The listing builds one solid part. Answer for the finished solid, in the listing's coordinates (mm). A direction names the side the tool comes from. Coordinates: 2 decimals unless noted, no trailing zeros. Order: outer loops, then holes, each group sorted by start corner. A loop starts at its lowest first (then second) coordinate and runs counter-clockwise, first axis right, second up.
from build123d import *

# Parameters (mm, degrees)
SKETCH007_W          = 124
SKETCH007_H          = 24.5
SKETCH007_R          = 2.5
PAD004_DEPTH         = 2
SKETCH006_R          = 3.175
PAD005_DEPTH         = 4.1125
PAD006_DEPTH         = 12.25
POCKET001_DEPTH      = 373.382623
POCKET001_DEPTH_BACK = 485.092667
PAD007_DEPTH         = 2
SKETCH011_W          = 35
SKETCH011_H          = 30
SKETCH011_W_2        = 15
SKETCH011_H_2        = 17
PAD008_DEPTH         = 12.25
HOLE_D               = 4.5
HOLE_CSINK_D         = 8.8
HOLE_CSINK_ANGLE     = 90
FILLET002_R          = 3
FILLET003_R          = 2
FILLET004_R          = 7
SKETCH017_W          = 3
SKETCH017_H          = 16.275
POCKET004_DEPTH      = 14.161
POCKET004_DEPTH_BACK = 213.001


with BuildPart() as part:
    # Sketch007 → Pad004 (new body)
    with BuildSketch(Plane.XZ.offset(13)):
        with Locations((78, 0)):
            Rectangle(SKETCH007_W, SKETCH007_H)
        with Locations((30, 0)):
            Circle(SKETCH007_R, mode=Mode.SUBTRACT)
        with BuildLine():
            ThreePointArc((90.8685, 2.143), (88.7255, 0), (90.8685, -2.143))
            Line((90.8685, -2.143), (98.806, -2.143))
            ThreePointArc((98.806, -2.143), (100.949, 0), (98.806, 2.143))
            Line((98.806, 2.143), (90.8685, 2.143))
        make_face(mode=Mode.SUBTRACT)
    extrude(amount=PAD004_DEPTH)

    # Sketch006 → Pad005 (join)
    with BuildSketch(Plane.XY.offset(12.25)):
        with BuildLine():
            Line((16, -13), (10.43, -13))
            Line((10.43, -13), (10.43, 3.73))
            ThreePointArc((10.43, 3.73), (2.257465, 13.912767), (-9.45279, 8.137908))
            ThreePointArc((-26.289956, 7.402782), (-17.64833, 2.661824), (-9.45279, 8.137908))
            Line((-26.289956, 7.402782), (-13.355703, -15))
            Line((-13.355703, -15), (16, -15))
            Line((16, -15), (16, -13))
        make_face()
        with Locations((0, 3.73)):
            Circle(SKETCH006_R, mode=Mode.SUBTRACT)
    pad005 = extrude(amount=-PAD005_DEPTH)

    # Mirrored001: Pad005 across XY
    add(pad005.mirror(Plane.XY))

    # Sketch008 → Pad006 (join, symmetric)
    with BuildSketch(Plane.XY):
        Polygon((-26.289956, 7.402782), (-28.289956, 9.134833), (-14.355703, -15), (-13.355703, -15), align=None)
    extrude(amount=PAD006_DEPTH, both=True)

    # Sketch009 → Pocket001 (cut, two sides)
    with BuildSketch(Plane.YZ) as pocket001_sk:
        with BuildLine():
            ThreePointArc((-13, 12.25), (-11.749286, 10.934524), (-10, 10.45))
            Line((-10, 10.45), (14.16, 10.45))
            Line((14.16, 12.25), (14.16, 10.45))
            Line((14.16, 12.25), (-13, 12.25))
        make_face()
    pocket001 = extrude(amount=-POCKET001_DEPTH, mode=Mode.SUBTRACT) + extrude(pocket001_sk.sketch, amount=POCKET001_DEPTH_BACK, mode=Mode.SUBTRACT)

    # Mirrored002: Pocket001 across Sketch009 H_Axis
    add(pocket001.mirror(Plane.XY), mode=Mode.SUBTRACT)

    # Sketch010 → Pad007 (join)
    with BuildSketch(Plane.XY.offset(12.25)):
        with BuildLine():
            Line((-13.355703, -15), (140, -15))
            Line((140, -15), (140, -45))
            Line((11.644297, -45), (140, -45))
            Line((16.00778, -59.929218), (11.644297, -45))
            Line((29.314371, -174.42131), (16.00778, -59.929218))
            Line((35.419102, -190.709129), (29.314371, -174.42131))
            Line((18.174297, -190.709129), (35.419102, -190.709129))
            ThreePointArc((18.174297, -190.709129), (11.242593, -193.580335), (8.371387, -200.512039))
            Line((8.371387, -210.497159), (8.371387, -200.512039))
            Line((-13.355703, -213), (8.371387, -210.497159))
            Line((-13.355703, -213), (-13.355703, -15))
        make_face()
    extrude(amount=-PAD007_DEPTH)

    # Sketch011 (on Face7 of Pad007) → Pad008 (join)
    with BuildSketch(Plane(origin=(0, 0, 12.25), x_dir=(-1, 0, 0), z_dir=(0, 0, 1))):
        with Locations((-36.144297, 30)):
            Rectangle(SKETCH011_W, SKETCH011_H)
        with Locations((-132.5, 36.5)):
            Rectangle(SKETCH011_W_2, SKETCH011_H_2)
        Polygon((13.355703, 174.42131), (-29.314371, 174.42131), (13.355703, 213), align=None)
    extrude(amount=-PAD008_DEPTH)

    # Hole (through all)
    with Locations(Plane.XY.offset(12.25)):
        with Locations((0, -190), (37.5, -30), (132.5, -36.5)):
            CounterSinkHole(HOLE_D / 2, HOLE_CSINK_D / 2, counter_sink_angle=HOLE_CSINK_ANGLE)

    # Fillet002
    fillet002_edges = [part.edges().sort_by_distance(p)[0] for p in [
        (96.822148, -15, 10.25),
    ]]
    fillet(fillet002_edges, radius=FILLET002_R)

    # Fillet003
    fillet003_edges = [part.edges().sort_by_distance(p)[0] for p in [
        (2.644297, -15, 10.25),
    ]]
    fillet(fillet003_edges, radius=FILLET003_R)

    # Fillet004
    fillet004_edges = [part.edges().sort_by_distance(p)[0] for p in [
        (125, -28, 5.125),
        (140, -45, 5.125),
    ]]
    fillet(fillet004_edges, radius=FILLET004_R)

    # Sketch017 → Pocket004 (cut, two sides)
    with BuildSketch(Plane.XZ) as pocket004_sk:
        with Locations((-14.855703, 0)):
            Rectangle(SKETCH017_W, SKETCH017_H)
    extrude(amount=-POCKET004_DEPTH, mode=Mode.SUBTRACT)
    extrude(pocket004_sk.sketch, amount=POCKET004_DEPTH_BACK, mode=Mode.SUBTRACT)


solid = part.part
1) Section B-B (y = -48) is taken. Give the vertices of the cut face in (x, z), then the cut area to 3 significant figures.
2) Section C-C (y = -74) is taken. Give the vertices of the cut face in (x, z).
3) Section A-A (x = 63) is taken. Give the vertices of the cut face in (y, z), then the cut area to 3 significant figures.
4) Consider L1, parallel to Y at x = 0, z = -9.45 (3 decimals); L2, parallel to Y at x = 37.5, z = 4.75; L3, parallel to Y at x = 0, z = 9.8 (3 decimals). Determine where each line is inside the solid, lowest interval first.
5) Determine the mould class of faces 6 (the face through (127.1, -30, 5.1)), 7 (the face through (137.9, -43, 6.2)), 8 (the face through (-4, -1, -10.45)) for opening direction Y: released by +Y, released by -Y, zero draft, split by the parting line, or undercut.
6) Each of these flat-tipped pins is pushed along its axis until it touches: P1, Ø0.6, axis at y = -14, z = -0.5, coming from the -X side; P2, Ø19.5, axis at x = 5.5, y = -191, coming from the -Z side; P3, Ø3, axis at x = 46, z = 1.5, coming from the -Y side. Where does it stop, or does it pass through?
7) A tool of negligible diameter and unlimited length cuts with its end or side. For faces 1 (the face through (36, -34, 0)), 2 (the face through (53.644, -30, 5)), 3 (the face through (136, -28, 5)), 4 (the face through (4, -95, 10.25)), 5 (the face through (-21.253, -1.321, 0.114)), from which of +Z, -Z, +X, -X, +Y, -Y can it reach the whole face along a straight path? Write none if from no direction.
Filled sheet:
1. outline: (-13.36, 10.25) - (12.52, 10.25) - (12.52, 12.25) - (-13.36, 12.25) - close
1. area: 51.8 mm2
2. outline: (-13.36, 10.25) - (17.64, 10.25) - (17.64, 12.25) - (-13.36, 12.25) - close
3. outline: (-45, 10.25) - (-18, 10.25) arc R3 cw to (-15, 7.25) - (-15, -12.25) - (-13, -12.25) - (-13, 12.25) - (-45, 12.25) - close
3. area: 111 mm2
4. L1: y = -15 to 0.555, 6.905 to 14.16
4. L2: y = -45 to -32.25, -27.75 to -13
4. L3: y = -200.925 to -192.25, -187.75 to -174.421, -15.736 to 0.555, 6.905 to 14.16
5. face 6: undercut
5. face 7: released by -Y
5. face 8: zero draft
6. P1: stops at x = 16
6. P2: stops at z = 0
6. P3: stops at y = -45
7. face 1: -Z, +X, -X, -Y
7. face 2: -Z, -Y
7. face 3: -Z, +X
7. face 4: -Z, -X
7. face 5: +X, +Y
